Here's how the part is built. I have some questions about the finished solid (model axes, mm). Face numbers are marked on the shaded views. Coordinates: 2 decimals unless noted, no trailing zeros. Order: outer loops, then holes, each group sorted by start corner. A loop starts at its lowest first (then second) coordinate and runs counter-clockwise, first axis right, second up. Notation, with made-up numbers: (19.25, -36) - (58.25, -36) arc R29 ccw to (58.25, 2) - close; hole circle Ø2 at (-38, 64). An arc over 180 degrees is marked (long way). Answer as CSV lines item,"result". Start each with the question number.
Q1. Suppose I cut it at D-D (z = 5). Count the separate pieces of the cut face and the enclosed holes in it, then the cut area to 3 significant figures.
Q2. Suppose I cut it at C-C (x = -14). Please give me the cut outline in (y, z).
Q3. Suppose I cut it at B-B (x = -45). Please give me the cut outline in (y, z).
Q4. Thinking about a two-plate mould opening in X: for the marked faces 1, 2, 3 and 4, which applies, released by +X, released by -X, zero draft, split by the parting line, or undercut?
Q5. Suppose I cut it at A-A (y = -2.5). Please give me the cut outline in (x, z).
Q6. I need wall thicknesses on line 1 (Z direction, x = 0, y = -11.25); line 2 (Z direction, x = -45, y = -9.25); line 3 (X direction, y = -18.25, z = -9). Which ranges of each line are inside material? Lowest first, please.
Q7. For pin 1 Ø6 at (x, y) = (4, -5.5) entering from +Z; pin 2 Ø1 at (y, z) = (-3.5, 6) entering from +X; pin 3 Ø12 at (x, y) = (-22.5, -4) entering from +Z, each with a flat end and sliding along its axis, tell me the tip position at first contact or that it passes through.
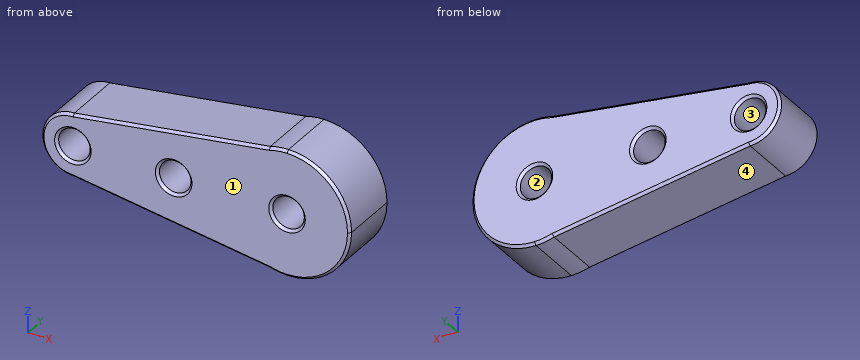
from build123d import *

# Parameters (mm, degrees)
F0_R     = 6.25
F1_DEPTH = 25
F2_SIZE  = 1
F3_SIZE  = 1


with BuildPart() as f1:
    # F0 (on Front) → F1 (new body)
    with BuildSketch(Plane.XZ):
        with BuildLine():
            ThreePointArc((0, -25), (17.67767, -17.67767), (25, 0))
            ThreePointArc((25, 0), (17.67767, 17.67767), (0, 25))
            Line((0, 25), (-7.19729, 23.941575))
            ThreePointArc((-7.19729, 23.941575), (-25, 0), (-7.19729, -23.941575))
            Line((-7.19729, -23.941575), (0, -25))
        make_face()
        Circle(F0_R, mode=Mode.SUBTRACT)
        with BuildLine():
            Line((-7.19729, 23.941575), (0, 25))
            ThreePointArc((0, 25), (-3.63735, 24.733978), (-7.19729, 23.941575))
        make_face()
        with BuildLine():
            ThreePointArc((-7.19729, -23.941575), (-3.63735, -24.733978), (0, -25))
            Line((0, -25), (-7.19729, -23.941575))
        make_face()
        with BuildLine():
            ThreePointArc((-7.19729, -23.941575), (-25, 0), (-7.19729, 23.941575))
            Line((-7.19729, 23.941575), (-85, 12.5))
            ThreePointArc((-85, 12.5), (-76.161165, 8.838835), (-72.5, 0))
            ThreePointArc((-72.5, 0), (-76.161165, -8.838835), (-85, -12.5))
            Line((-85, -12.5), (-7.19729, -23.941575))
        make_face()
        with Locations((-45, 0)):
            Circle(F0_R, mode=Mode.SUBTRACT)
        with BuildLine():
            ThreePointArc((-72.5, 0), (-76.161165, 8.838835), (-85, 12.5))
            ThreePointArc((-85, 12.5), (-97.5, 0), (-85, -12.5))
            ThreePointArc((-85, -12.5), (-76.161165, -8.838835), (-72.5, 0))
        make_face()
        with Locations((-85, 0)):
            Circle(F0_R, mode=Mode.SUBTRACT)
    extrude(amount=F1_DEPTH)

    # F2
    f2_edges = [f1.edges().sort_by_distance(p)[0] for p in [
        (-3.63735, -25, 24.733978),
        (-46.098645, -25, 18.220787),
        (-97.5, -25, 0),
        (-46.098645, -25, -18.220787),
        (24.733978, -25, -3.63735),
        (-6.25, -25, 0),
        (-51.25, -25, 0),
        (-91.25, -25, 0),
    ]]
    chamfer(f2_edges, length=F2_SIZE)

    # F3
    f3_edges = [f1.edges().sort_by_distance(p)[0] for p in [
        (-3.63735, 0, 24.733978),
        (-46.098645, 0, 18.220787),
        (-97.5, 0, 0),
        (-46.098645, 0, -18.220787),
        (24.733978, 0, -3.63735),
        (-6.25, 0, 0),
        (-51.25, 0, 0),
        (-91.25, 0, 0),
    ]]
    chamfer(f3_edges, length=F3_SIZE)


solid = f1.part
Here are the results:
1,separate pieces,"4"
1,enclosed holes,"0"
1,area,"2,450 mm²"
2,outline,"(-25, -21.93) - (-24, -22.94) - (-1, -22.94) - (0, -21.93) - (0, 21.93) - (-1, 22.94) - (-24, 22.94) - (-25, 21.93) - close"
3,outline,"(-25, -17.37) - (-24, -18.38) - (-1, -18.38) - (0, -17.37) - (0, -7.25) - (-1, -6.25) - (-24, -6.25) - (-25, -7.25) - close; (-25, 7.25) - (-24, 6.25) - (-1, 6.25) - (0, 7.25) - (0, 17.37) - (-1, 18.38) - (-24, 18.38) - (-25, 17.37) - close"
4,face 1,"zero draft"
4,face 2,"undercut"
4,face 3,"undercut"
4,face 4,"released by -X"
5,outline,"(-85, -12.5) - (-7.2, -23.94) arc R25 ccw to (0, -25) arc R25 ccw to (25, 0) arc R25 ccw to (0, 25) arc R25 ccw to (-7.2, 23.94) - (-85, 12.5) arc R12.5 ccw to start; hole circle Ø12.5 at (-85, 0); hole circle Ø12.5 at (-45, 0); hole circle Ø12.5 at (0, 0)"
6,line 1,"z = -25 to -6.25, 6.25 to 25"
6,line 2,"z = -18.38 to -6.25, 6.25 to 18.38"
6,line 3,"x = -93.67 to 23.32"
7,pin 1,"stops at z = 24.98"
7,pin 2,"stops at x = 24.39"
7,pin 3,"stops at z = 22.57"
